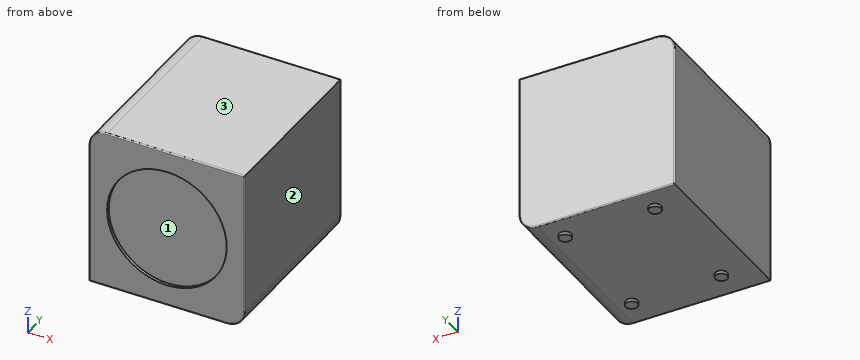
```python
from build123d import *

# Parameters (mm, degrees)
F1_DEPTH = 290
F2_R     = 10
F3_DEPTH = 5
F4_R     = 2
F5_R     = 100
F6_DEPTH = 5


with BuildPart() as f1:
    # F0 (on Front) → F1 (new body)
    with BuildSketch(Plane.XZ):
        with BuildLine():
            Line((-130, -135), (100, -135))
            ThreePointArc((100, -135), (121.213203, -126.213203), (130, -105))
            Line((130, -105), (130, 135))
            Line((130, 135), (-100, 135))
            ThreePointArc((-100, 135), (-121.213203, 126.213203), (-130, 105))
            Line((-130, 105), (-130, -135))
        make_face()
    extrude(amount=-F1_DEPTH)

    # F2 (on face) → F3 (join)
    with BuildSketch(Plane(origin=(0, 0, -135), x_dir=(1, 0, 0), z_dir=(0, 0, -1))):
        with Locations((-75, -50)):
            Circle(F2_R)
        with Locations((75, -50)):
            Circle(F2_R)
        with Locations((75, -250)):
            Circle(F2_R)
        with Locations((-75, -250)):
            Circle(F2_R)
    extrude(amount=F3_DEPTH)

    # F4
    f4_edges = [f1.edges().sort_by_distance(p)[0] for p in [
        (-15, 0, -135),
        (121.213203, 0, -126.213203),
        (130, 0, 15),
        (15, 0, 135),
        (-121.213203, 0, 126.213203),
        (-130, 0, -15),
        (-15, 290, -135),
        (121.213203, 290, -126.213203),
        (130, 290, 15),
        (15, 290, 135),
        (-121.213203, 290, 126.213203),
        (-130, 290, -15),
    ]]
    fillet(f4_edges, radius=F4_R)

    # F5 (on face) → F6 (cut)
    with BuildSketch(Plane.XZ):
        Circle(F5_R)
    extrude(amount=-F6_DEPTH, mode=Mode.SUBTRACT)


solid = f1.part
```
Work out the finished part from the listing and answer in its coordinate system (mm). Face numbers are marked on the shaded views. Coordinates: 2 decimals unless noted, no trailing zeros. Write each loop counter-clockwise with the first axis right and the second up, starting at its lowest first coordinate (ties: lowest second). Pieces come first, ordered by that corner, then holes. Notation, with made-up numbers: (33, 53.5) - (69, 53.5) arc R28 cw to (69, 89.5) - close; hole circle Ø1 at (-6.75, 83). An arc over 180 degrees is marked (long way). Answer as a JSON object with one key per item and string values.
Q1. Find section D-D (x = 72.5). Write down the section's boundary in (y, z), plus the area to 3 significant figures.
Results list:
{"outline": "(0, -133) arc R2 ccw to (2, -135) - (40.32, -135) - (40.32, -140) - (59.68, -140) - (59.68, -135) - (240.32, -135) - (240.32, -140) - (259.68, -140) - (259.68, -135) - (288, -135) arc R2 ccw to (290, -133) - (290, 133) arc R2 ccw to (288, 135) - (2, 135) arc R2 ccw to (0, 133) - (0, 68.87) - (5, 68.87) - (5, -68.87) - (0, -68.87) - close", "area": "77,800 mm^2"}
Q2. Given pin 1 Ø12 at (x, y) = (-9.5, 218) entering from -Z; pin 2 Ø8 at (x, z) = (49.5, -79) entering from -Y, each flat-ended and moving along its own axis, determine where each tip first touches the part or whether it passes through.
Results list:
{"pin 1": "stops at z = -135", "pin 2": "stops at y = 5"}
Q3. For a pull along X with two mould halves and no side action, classify the marked faces 1, 2 and 3 as pulls with the +X half, pulls with the -X half, needs draft (parallel to the pull), parting line crosses it, or undercut.
Results list:
{"face 1": "undercut", "face 2": "pulls with the +X half", "face 3": "needs draft"}
Q4. Find section B-B (x = 0). Write down the section's boundary in (y, z).
Results list:
{"outline": "(0, -133) arc R2 ccw to (2, -135) - (288, -135) arc R2 ccw to (290, -133) - (290, 133) arc R2 ccw to (288, 135) - (2, 135) arc R2 ccw to (0, 133) - (0, 100) - (5, 100) - (5, -100) - (0, -100) - close"}
Q5. Find section A-A (y = 250). Write down the section's boundary in (x, z).
Results list:
{"outline": "(-130, -135) - (-85, -135) - (-85, -140) - (-65, -140) - (-65, -135) - (65, -135) - (65, -140) - (85, -140) - (85, -135) - (100, -135) arc R30 ccw to (130, -105) - (130, 135) - (-100, 135) arc R30 ccw to (-130, 105) - close"}
Q6. Find section C-C (y = 111.5). Write down the section's boundary in (x, z).
Results list:
{"outline": "(-130, -135) - (100, -135) arc R30 ccw to (130, -105) - (130, 135) - (-100, 135) arc R30 ccw to (-130, 105) - close"}
Q7. Consider L1, parallel to Z at x = 0, y = 3.05; L2, parallel to X at y = 123, z = -106; L3, parallel to Y at x = 67.5, z = 49. Determine where each line is inside the solid, lowest interval first. Write a range as from..to.
Results list:
{"L1": "z = -135..-100, 100..135", "L2": "x = -130..129.98", "L3": "y = 5..290"}
